Work out the finished part from the listing and answer in its coordinate system (mm). Coordinates: 2 decimals unless noted, no trailing zeros. Order: outer loops, then holes, each group sorted by start corner. A loop starts at its lowest first (then second) coordinate and runs counter-clockwise, first axis right, second up. Notation, with made-up numbers: M 30.25,-5.5 L 40.25,-5.5 A21 cw 40.25,21.5 Z; hole C 18,-14 d1. An arc over 180 degrees is marked long. Answer in a Markdown table with one row per item. Add a question column.
Item 1: The part is cut by section A-A (y = -29.5). Write down the section's boundary in (x, z), then the cut area to 3 significant figures.
Item 2: Consider line 1 (Y direction, x = 322, z = 4.3); line 2 (X direction, y = -167, z = 0.7); line 3 (Y direction, x = 129.5, z = 4.5). Determine where each line is inside the solid, lowest interval first. Write a range as from..to.
Item 3: Flat-ended cylindrical pins translate along their axes: pin 1 Ø0.8 at (y, z) = (-103.5, 2.5) entering from +X; pin 2 Ø3 at (x, z) = (346.5, 4) entering from +Y; pin 3 Ø1 at (x, z) = (312.5, 4) entering from +Y. Find the tip coordinate at first contact, or state that the pin passes through.
Item 4: The part is cut by section B-B (x = 298). Write down the section's boundary in (y, z).
from build123d import *

# Parameters (mm, degrees)
BOSS_EXTRUDE1_DEPTH = 6


with BuildPart() as part:
    # Sketch1 → Boss-Extrude1 (new body)
    with BuildSketch(Plane.XY):
        with BuildLine():
            Line((-6, 0), (-6, -494.15))
            ThreePointArc((-6, -494.15), (-4.242640687, -498.392640687), (0, -500.15))
            Line((0, -500.15), (402, -500.15))
            ThreePointArc((402, -500.15), (406.242640687, -498.392640687), (408, -494.15))
            Line((408, -494.15), (408, -119.649819196))
            ThreePointArc((408, -119.649819196), (406.242640687, -115.407178509), (402, -113.649819196))
            Line((402, -113.649819196), (344.227783268, -113.649819196))
            ThreePointArc((344.227783268, -113.649819196), (338.727783268, -108.149819196), (344.227783268, -102.649819196))
            Line((344.227783268, -102.649819196), (351.727783268, -102.649819196))
            Line((351.727783268, -102.649819196), (351.727783268, -104.149819196))
            Line((351.727783268, -104.149819196), (344.227783268, -104.149819196))
            ThreePointArc((344.227783268, -104.149819196), (340.227783268, -108.149819196), (344.227783268, -112.149819196))
            Line((344.227783268, -112.149819196), (402, -112.149819196))
            ThreePointArc((402, -112.149819196), (407.303300859, -114.346518337), (409.5, -119.649819196))
            Line((409.5, -119.649819196), (409.5, -494.15))
            ThreePointArc((409.5, -494.15), (407.303300859, -499.453300859), (402, -501.65))
            Line((402, -501.65), (0, -501.65))
            ThreePointArc((0, -501.65), (-5.303300859, -499.453300859), (-7.5, -494.15))
            Line((-7.5, -494.15), (-7.5, 0))
            ThreePointArc((-7.5, 0), (0, 7.5), (7.5, 0))
            Line((7.5, 0), (7.5, -106.149819196))
            ThreePointArc((7.5, -106.149819196), (9.257359313, -110.392459883), (13.5, -112.149819196))
            Line((13.5, -112.149819196), (325.227783268, -112.149819196))
            ThreePointArc((325.227783268, -112.149819196), (329.227783268, -108.149819196), (325.227783268, -104.149819196))
            Line((325.227783268, -104.149819196), (317.727783268, -104.149819196))
            Line((317.727783268, -104.149819196), (317.727783268, -102.649819196))
            Line((317.727783268, -102.649819196), (325.227783268, -102.649819196))
            ThreePointArc((325.227783268, -102.649819196), (330.727783268, -108.149819196), (325.227783268, -113.649819196))
            Line((325.227783268, -113.649819196), (13.5, -113.649819196))
            ThreePointArc((13.5, -113.649819196), (8.196699141, -111.453120055), (6, -106.149819196))
            Line((6, -106.149819196), (6, 0))
            ThreePointArc((6, 0), (0, 6), (-6, 0))
        make_face()
    extrude(amount=BOSS_EXTRUDE1_DEPTH)


solid = part.part
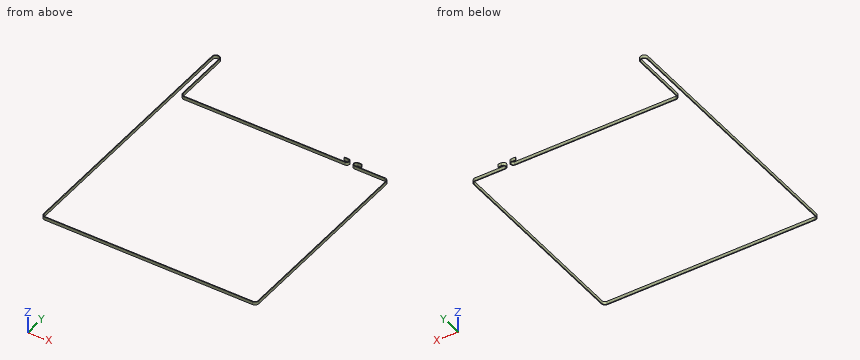
Reply:
| question | item | result |
|---|---|---|
| 1 | outline | M -7.5,0 L -6,0 L -6,6 L -7.5,6 Z; M 6,0 L 7.5,0 L 7.5,6 L 6,6 Z |
| 1 | area | 18.0 mm2 |
| 2 | line 1 | y = -501.65..-500.15, -113.65..-112.15, -104.15..-102.65 |
| 2 | line 2 | x = -7.5..-6, 408..409.5 |
| 2 | line 3 | y = -501.65..-500.15, -113.65..-112.15 |
| 3 | pin 1 | stops at x = 351.73 |
| 3 | pin 2 | stops at y = -102.65 |
| 3 | pin 3 | stops at y = -112.15 |
| 4 | outline | M -501.65,0 L -500.15,0 L -500.15,6 L -501.65,6 Z; M -113.65,0 L -112.15,0 L -112.15,6 L -113.65,6 Z |
